Work out the finished part from the listing and answer in its coordinate system (mm). A direction names the side the tool comes from. Give positions to 0.01 mm unless a question says otherwise; leave off trailing zeros. Loops run counter-clockwise (first coordinate to the right, second up) from the corner with the lowest first, then second, coordinate; pieces in that order, holes last. Notation, with made-up numbers: M -23,18 L -12,18 A11 cw -12,24 Z; hole C 12.5,18.5 d10. An arc over 180 degrees is marked long. Write item = value, one per line. Start each with the question number.
1. Section A-A on y = 6 is taken. Determine the outline of the cut face in (x, z).
2. Flat-ended cylindrical pins translate along their axes: pin 1 Ø1 at (x, y) = (10.5, 1.5) entering from +Z; pin 2 Ø12 at (x, z) = (26, 5.5) entering from +Y; pin 3 Ø4 at (x, z) = (6.5, 13) entering from +Y; pin 4 Ø5 at (x, y) = (20.5, 8) entering from +Z. Find the tip coordinate at first contact, or state that the pin passes through.
3. Consider L1, parallel to X at y = 9.75, z = 2.5; L2, parallel to X at y = 2.5, z = 4; L3, parallel to Y at x = 8.5, z = 1.5. Determine where each line is inside the solid, lowest interval first. Write a range as [from, to].
4. For faces 5 (the face through (18, 1, 40)), 6 (the face through (12, 1, 0)), 7 (the face through (15, 0, 20)), 8 (the face through (3, 3, 1)), determine the directions among +Z, -Z, +X, -X, +Y, -Y from which every point of the face is accessible in a straight line to the end or side of a thin tool.
5. Section B-B on z = 33 is taken. Determine the outline of the cut face in (x, y).
6. Section D-D on x = 25 is taken. Determine the outline of the cut face in (y, z).
7. Section C-C on z = 41.5 is taken. Determine the outline of the cut face in (x, y), plus the area to 3 significant figures.
8. The mould has two halves that part along X. Classify faces 1 (the face through (30, 1, 23)), 2 (the face through (25, 10, 2)), 3 (the face through (0, 1, 17)), 4 (the face through (7.48, 3.48, 32.67)): released by +X, released by -X, zero draft, split by the parting line, or undercut.
```python
from build123d import *

# Parameters (mm, degrees)
SKETCH1_R           = 2.15
BOSS_EXTRUDE1_DEPTH = 2
SKETCH2_R           = 1.5
BOSS_EXTRUDE2_DEPTH = 10
SKETCH3_R           = 2.5
BOSS_EXTRUDE3_DEPTH = 5


with BuildPart() as part:
    # Sketch1 → Boss-Extrude1 (new body)
    with BuildSketch(Plane(origin=(0, 0, 0), x_dir=(1, 0, 0), z_dir=(0, 1, 0))):
        with BuildLine():
            Line((24.343145751, 0), (0, 0))
            Line((0, 0), (0, -34.343145751))
            Line((0, -34.343145751), (-5.656854249, -40))
            ThreePointArc((-5.656854249, -40), (-5.656854249, -45.656854249), (0, -45.656854249))
            Line((0, -45.656854249), (5.656854249, -40))
            Line((5.656854249, -40), (30, -40))
            Line((30, -40), (30, -5.656854249))
            Line((30, -5.656854249), (35.656854249, 0))
            ThreePointArc((35.656854249, 0), (35.656854249, 5.656854249), (30, 5.656854249))
            Line((30, 5.656854249), (24.343145751, 0))
        make_face()
        with Locations(Location((32.828427125, 2.828427125, 0), (0, 0, 270))):
            Circle(SKETCH1_R, mode=Mode.SUBTRACT)
        with Locations(Location((-2.828427125, -42.828427125, 0), (0, 0, 270))):
            Circle(SKETCH1_R, mode=Mode.SUBTRACT)
    extrude(amount=BOSS_EXTRUDE1_DEPTH)

    # Sketch2 → Boss-Extrude2 (add)
    with BuildSketch(Plane(origin=(0, 0, 0), x_dir=(1, 0, 0), z_dir=(0, 1, 0))):
        with Locations(Location((25, -2.5, 0), (0, 0, 270))):
            Circle(SKETCH2_R)
        with Locations(Location((25, -33, 0), (0, 0, 270))):
            Circle(SKETCH2_R)
        with Locations(Location((5, -33, 0), (0, 0, 270))):
            Circle(SKETCH2_R)
        with Locations(Location((5, -2.5, 0), (0, 0, 270))):
            Circle(SKETCH2_R)
    extrude(amount=BOSS_EXTRUDE2_DEPTH)

    # Sketch3 → Boss-Extrude3 (add)
    with BuildSketch(Plane(origin=(0, 0, 0), x_dir=(1, 0, 0), z_dir=(0, 1, 0))):
        with Locations(Location((5, -2.5, 0), (0, 0, 90))):
            Circle(SKETCH3_R)
        with Locations(Location((25, -2.5, 0), (0, 0, 270))):
            Circle(SKETCH3_R)
        with Locations(Location((25, -33, 0), (0, 0, 270))):
            Circle(SKETCH3_R)
        with Locations(Location((5, -33, 0), (0, 0, 270))):
            Circle(SKETCH3_R)
    extrude(amount=BOSS_EXTRUDE3_DEPTH)


solid = part.part
```
Verdict:
q1.outline = C 5,2.5 d3; C 5,33 d3; C 25,2.5 d3; C 25,33 d3
q2.pin_1 = 40
q2.pin_2 = 10
q2.pin_3 = 2
q2.pin_4 = through
q3.L1 = [3.5, 6.5], [23.5, 26.5]
q3.L2 = [3, 7], [23, 27]
q3.L3 = [0, 2]
q4.face_5 = +Z, +X, +Y, -Y
q4.face_6 = -Z, -X, +Y, -Y
q4.face_7 = +Z, -Z, +X, -X, -Y
q4.face_8 = +Y
q5.outline = M 0,0 L 30,0 L 30,2 L 27.5,2 L 27.5,5 L 26.5,5 L 26.5,10 L 23.5,10 L 23.5,5 L 22.5,5 L 22.5,2 L 7.5,2 L 7.5,5 L 6.5,5 L 6.5,10 L 3.5,10 L 3.5,5 L 2.5,5 L 2.5,2 L 0,2 Z
q6.outline = M 0,-0.66 L 2,-0.66 L 2,0 L 5,0 L 5,1 L 10,1 L 10,4 L 5,4 L 5,5 L 2,5 L 2,30.5 L 5,30.5 L 5,31.5 L 10,31.5 L 10,34.5 L 5,34.5 L 5,35.5 L 2,35.5 L 2,40 L 0,40 Z
q7.outline = M -6.6,0 L -4.52,0 L -4.52,2 L -6.6,2 Z; M -1.14,0 L 4.16,0 L 4.16,2 L -1.14,2 Z
q7.area = 14.8 mm2
q8.face_1 = released by +X
q8.face_2 = zero draft
q8.face_3 = released by -X
q8.face_4 = undercut
